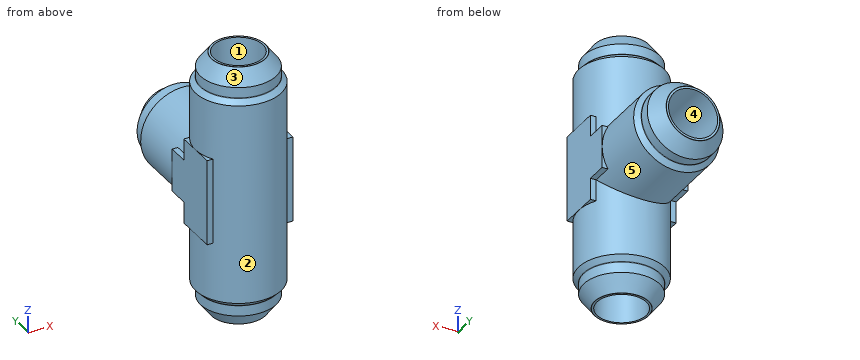
```python
from build123d import *

# Parameters (mm, degrees)
SKETCH4_W           = 19.3294
SKETCH4_H           = 13.49375
CIRPATTERN1_COUNT   = 3
CIRPATTERN1_ANGLE   = 180
BOSS_EXTRUDE1_DEPTH = 13.49375
CIRPATTERN2_COUNT   = 3
CIRPATTERN2_ANGLE   = 180


with BuildPart() as part:
    # Sketch1 → Revolve1 (revolve)
    with BuildSketch(Plane(origin=(0, 0, 0), x_dir=(0, 0, -1), z_dir=(1, 0, 0))):
        with BuildLine():
            Line((-41.275, 0), (-19.3294, 0))
            Line((-19.3294, 0), (-19.3294, 12.0015))
            Line((-19.3294, 12.0015), (-19.3294, 13.49375))
            Line((-19.3294, 13.49375), (-23.99665, 13.49375))
            Line((-23.99665, 13.49375), (-31.69285, 13.49375))
            Line((-31.69285, 13.49375), (-33.199605122, 11.986994878))
            ThreePointArc((-33.199605122, 11.986994878), (-33.282008653, 11.931934599), (-33.379210245, 11.9126))
            Line((-33.379210245, 11.9126), (-36.65714943, 11.9126))
            Line((-36.65714943, 11.9126), (-41.224430508, 8.470906846))
            ThreePointArc((-41.224430508, 8.470906846), (-41.261656664, 8.426147258), (-41.275, 8.369480136))
            Line((-41.275, 8.369480136), (-41.275, 0))
        make_face()
    revolve(axis=Axis((0, 0, 19.812), (0, 0, -1)))

    # Sketch4 → Revolve2 (revolve)
    with BuildSketch(Plane(origin=(0, 0, 0), x_dir=(0, 0, -1), z_dir=(1, 0, 0))):
        with Locations((-9.6647, 6.746875)):
            Rectangle(SKETCH4_W, SKETCH4_H)
    revolve(axis=Axis((0, 0, 0), (0, 0, 1)))


with BuildPart() as cirpattern1_1:
    # CirPattern1: pattern copy
    add(part.part.rotate(Axis((0, 0, 0), (-1, 0, 0)), 1 * CIRPATTERN1_ANGLE / (CIRPATTERN1_COUNT - 1)))


with BuildPart() as cirpattern1_2:
    # CirPattern1: pattern copy
    add(part.part.rotate(Axis((0, 0, 0), (-1, 0, 0)), 2 * CIRPATTERN1_ANGLE / (CIRPATTERN1_COUNT - 1)))


with BuildPart() as cirpattern1_1_1:
    add(cirpattern1_1.part)

    # Combine1: union CirPattern1_2, part
    add(cirpattern1_2.part)
    add(part.part)

    # Sketch5 → Boss-Extrude1 (add, symmetric)
    with BuildSketch(Plane(origin=(0, 0, 0), x_dir=(0, 0, -1), z_dir=(1, 0, 0))):
        Polygon((-6.746875, 13.49375), (6.746875, 13.49375), (6.746875, 6.746875), (13.49375, 6.746875), (13.49375, -6.746875), (-13.49375, -6.746875), (-13.49375, 6.746875), (-6.746875, 6.746875), align=None)
    extrude(amount=BOSS_EXTRUDE1_DEPTH, both=True)

    # Sketch6 → Cut-Revolve1 (revolve, cut)
    with BuildSketch(Plane(origin=(0, 0, 0), x_dir=(0, 0, -1), z_dir=(1, 0, 0))):
        with BuildLine():
            Line((-41.275, 7.7343), (0, 7.7343))
            ThreePointArc((0, 7.7343), (5.468975978, 5.468975978), (7.7343, 0))
            Line((7.7343, 0), (-41.275, 0))
            Line((-41.275, 0), (-41.275, 7.7343))
        make_face()
    cut_revolve1 = revolve(axis=Axis((0, 0, -7.7343), (0, 0, 1)), mode=Mode.SUBTRACT)

    # CirPattern2: Cut-Revolve1 ×3 about axis
    cirpattern2_axis = Axis((-10.773895932, 0, 0), (-1, 0, 0))
    for i in range(1, CIRPATTERN2_COUNT):
        add(cut_revolve1.rotate(cirpattern2_axis, i * CIRPATTERN2_ANGLE / (CIRPATTERN2_COUNT - 1)), mode=Mode.SUBTRACT)


solid = cirpattern1_1_1.part
```
Could you check a few things on this model? Use its own coordinates, in mm. Face numbers are marked on the shaded views. A direction names the side the tool comes from. Coordinates: 2 decimals unless noted, no trailing zeros. Loops run counter-clockwise (first coordinate to the right, second up) from the corner with the lowest first, then second, coordinate; pieces in that order, holes last.
1) Imagine slicing it at B-B (z = -24.5). List the corners of the cut face in (x, y) for me.
Reported:
outline: circle Ø26.99 at (0, 0); hole circle Ø15.47 at (0, 0)
2) Thinking about a two-plate mould opening in Z: for the marked faces 3, 4 and 5, which applies, released by +Z, released by -Z, zero draft, split by the parting line, or undercut?
Reported:
face 3: released by +Z
face 4: undercut
face 5: split by the parting line
3) Which directions (+Z, -Z, +X, -X, +Y, -Y) give clear straight access to the entire face, cutting with the end or side of a thin tool? Please do the marked faces 1 and 2.
Reported:
face 1: +Z, -Z
face 2: none
4) Will these pins go through, and if not, where does the flat tip stop? pin 1 Ø6 at (y, z) = (16.5, 14.5) entering from +X; pin 2 Ø4 at (y, z) = (25, -7) entering from +X; pin 3 Ø10 at (y, z) = (-6.5, 19) entering from -X.
Reported:
pin 1: stops at x = 7.06
pin 2: stops at x = 12.53
pin 3: stops at x = -13.41
5) Please list where this line runs through material, in increasing order: line 1 along X through (y, z) = (22.5, 0).
Reported:
line 1: x = -13.49 to -7.73, 7.73 to 13.49
6) Imagine slicing it at A-A (x = 0). State how many separate pieces and enclosed holes the cut face has, and give its area (3 significant figures).
Reported:
separate pieces: 3
enclosed holes: 0
area: 1,050 mm2
